Could you check a few things on this model? Use its own coordinates, in mm. Face numbers are marked on the shaded views. A direction names the side the tool comes from. Round coordinates to 2 decimals unless told otherwise and drop trailing zeros. Write each loop counter-clockwise with the first axis right and the second up, starting at its lowest first coordinate (ties: lowest second). Pieces come first, ordered by that corner, then holes. Notation, with made-up numbers: (48, 87.5) -> (102, 87.5) arc R13 ccw to (102, 105.5) -> close; hole circle Ø8 at (44, -27). An arc over 180 degrees is marked (long way). Answer as CSV lines item,"result". Start each with the question number.
Q1. Imagine slicing it at C-C on y = -17. Please give me the cut outline in (x, z), and give its area (3 significant figures).
Q2. Imagine slicing it at B-B on x = 4.5. Please give me the cut outline in (y, z).
Q3. If we mould it in two halves opening along Y, with no side actions, what happens to the marked faces 3, 4 and 5? For each: pulls with the +Y half, pulls with the -Y half, needs draft (parallel to the pull), parting line crosses it, or undercut.
Q4. If I drill on line 1 (X direction, y = -11, z = 2.4); line 2 (Y direction, x = -5, z = 2.25); line 3 (Y direction, x = 7.25, z = 0.7), over which ranges is the centre line in solid material (lowest first)? Write a range as [from, to].
Q5. For the marked faces 1 and 2, which set-ups out of +Z, -Z, +X, -X, +Y, -Y let a thin tool reach every point of the face, with its end or its side?
Q6. Imagine slicing it at D-D on x = -5.5. Please give me the cut outline in (y, z), and give its area (3 significant figures).
Q7. Imagine slicing it at A-A on y = -12.75. Please give me the cut outline in (x, z), and give its area (3 significant figures).
Q8. Will these pins go through, and if not, where does the flat tip stop? pin 1 Ø1 at (x, z) = (2, 1.5) entering from +Y; pin 2 Ø1.2 at (y, z) = (-18.5, 0.5) entering from +X; pin 3 Ø1.2 at (y, z) = (-17.5, 1.5) entering from -X.
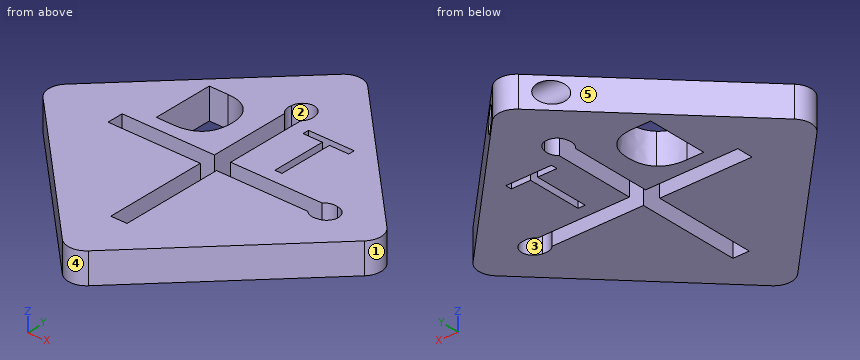
from build123d import *

# Parameters (mm, degrees)
F1_DEPTH = 2.5
F2_R     = 0.85
F3_DEPTH = 12.5


with BuildPart() as f1:
    # F0 (on Top) → F1 (new body)
    with BuildSketch(Plane.XY):
        with BuildLine():
            Line((13.081475452, -13.081475452), (1.0606601718, -1.0606601718))
            ThreePointArc((1.0606601718, -1.0606601718), (0, -0.6213203436), (-1.0606601718, -1.0606601718))
            Line((-1.0606601718, -1.0606601718), (-13.081475452, -13.081475452))
            ThreePointArc((-13.081475452, -13.081475452), (-13.5208152802, -14.1421356237), (-13.081475452, -15.2027957955))
            Line((-13.081475452, -15.2027957955), (-1.0606601718, -27.2236110757))
            ThreePointArc((-1.0606601718, -27.2236110757), (0, -27.6629509039), (1.0606601718, -27.2236110757))
            Line((1.0606601718, -27.2236110757), (13.081475452, -15.2027957955))
            ThreePointArc((13.081475452, -15.2027957955), (13.5208152802, -14.1421356237), (13.081475452, -13.081475452))
        make_face()
        with BuildLine():
            add(Edge.make_bspline(
                [(-2.95422167, -8.1059920208), (-2.3134881631, -8.7467255278), (-2.3134881631, -9.8968991389)],
                knots=[0, 0, 0, 1, 1, 1], degree=2))
            add(Edge.make_bspline(
                [(-2.3134881631, -9.8968991389), (-2.3134881631, -11.1241126806), (-2.9797208019, -11.7735267431)],
                knots=[0, 0, 0, 1, 1, 1], degree=2))
            add(Edge.make_bspline(
                [(-2.9797208019, -11.7735267431), (-3.6459534408, -12.4229408056), (-4.8970385103, -12.4229408056)],
                knots=[0, 0, 0, 1, 1, 1], degree=2))
            Line((-4.8970385103, -12.4229408056), (-6.2707364269, -12.4229408056))
            Line((-6.2707364269, -12.4229408056), (-6.2707364269, -7.4652585139))
            Line((-6.2707364269, -7.4652585139), (-4.7516392047, -7.4652585139))
            add(Edge.make_bspline(
                [(-4.7516392047, -7.4652585139), (-3.5949551769, -7.4652585139), (-2.95422167, -8.1059920208)],
                knots=[0, 0, 0, 1, 1, 1], degree=2))
        make_face(mode=Mode.SUBTRACT)
        with BuildLine():
            Line((-8.1334756687, -14.8039748892), (-8.1334756687, -13.4802963582))
            Line((-8.1334756687, -13.4802963582), (-0.6236797201, -13.4802963582))
            Line((-0.6236797201, -13.4802963582), (-0.6236797201, -6.9198086858))
            ThreePointArc((-0.6236797201, -6.9198086858), (-0.9032194318, -6.4583786209), (-0.9135835525, -5.9189782686))
            ThreePointArc((-0.9135835525, -5.9189782686), (0.0168397474, -5.0141534426), (0.9868078824, -5.876451129))
            ThreePointArc((0.9868078824, -5.876451129), (0.9900106564, -6.4384308628), (0.6999988109, -6.9198086858))
            Line((0.6999988109, -6.9198086858), (0.6999988109, -13.4802963582))
            Line((0.6999988109, -13.4802963582), (8.1334756687, -13.4802963582))
            ThreePointArc((8.1334756687, -13.4802963582), (8.5949057336, -13.2007566465), (9.134306086, -13.1903925258))
            ThreePointArc((9.134306086, -13.1903925258), (10.0391309119, -14.1208158258), (9.1768332255, -15.0907839607))
            ThreePointArc((9.1768332255, -15.0907839607), (8.6148534917, -15.0939867347), (8.1334756687, -14.8039748892))
            Line((8.1334756687, -14.8039748892), (0.6999988109, -14.8039748892))
            Line((0.6999988109, -14.8039748892), (0.6999988109, -23.1867600232))
            Line((0.6999988109, -23.1867600232), (-0.6236797201, -23.1867600232))
            Line((-0.6236797201, -23.1867600232), (-0.6236797201, -14.8039748892))
            Line((-0.6236797201, -14.8039748892), (-8.1334756687, -14.8039748892))
        make_face(mode=Mode.SUBTRACT)
        Polygon((3.9598674141, -7.9774117573), (3.9598674141, -12.4229412712), (3.3836955391, -12.4229412712), (3.3836955391, -7.9774117573), (1.813600053, -7.9774117573), (1.813600053, -7.4652589795), (5.5299629002, -7.4652589795), (5.5299629002, -7.9774117573), align=None, mode=Mode.SUBTRACT)
    extrude(amount=F1_DEPTH)

    # F2 (on Right) → F3 (cut, symmetric)
    with BuildSketch(Plane.YZ):
        with Locations((-2.4908210296, 1.292226194)):
            Circle(F2_R)
    extrude(amount=F3_DEPTH, both=True, mode=Mode.SUBTRACT)


solid = f1.part
Checks:
1,outline,"(-11.28, 0) -> (-0.62, 0) -> (-0.62, 2.5) -> (-11.28, 2.5) -> close; (0.7, 0) -> (11.28, 0) -> (11.28, 2.5) -> (0.7, 2.5) -> close"
1,area,"53.1 mm^2"
2,outline,"(-23.78, 0) -> (-14.8, 0) -> (-14.8, 2.5) -> (-23.78, 2.5) -> close; (-13.48, 0) -> (-7.98, 0) -> (-7.98, 2.5) -> (-13.48, 2.5) -> close; (-7.47, 0) -> (-4.5, 0) -> (-4.5, 2.5) -> (-7.47, 2.5) -> close"
3,face 3,"undercut"
3,face 4,"pulls with the -Y half"
3,face 5,"pulls with the +Y half"
4,line 1,"[-11, -6.27], [-2.49, -0.62], [0.7, 3.38], [3.96, 11]"
4,line 2,"[-23.28, -14.8], [-13.48, -12.42], [-7.47, -5]"
4,line 3,"[-21.03, -14.8], [-13.48, -7.25]"
5,face 1,"+Z, -Z, +X"
5,face 2,"+Z, -Z"
6,outline,"(-22.78, 0) -> (-14.8, 0) -> (-14.8, 2.5) -> (-22.78, 2.5) -> close; (-13.48, 0) -> (-12.42, 0) -> (-12.42, 2.5) -> (-13.48, 2.5) -> close; (-7.47, 0) -> (-5.5, 0) -> (-5.5, 2.5) -> (-7.47, 2.5) -> close"
6,area,"27.5 mm^2"
7,outline,"(-12.75, 0) -> (-0.62, 0) -> (-0.62, 2.5) -> (-12.75, 2.5) -> close; (0.7, 0) -> (12.75, 0) -> (12.75, 2.5) -> (0.7, 2.5) -> close"
7,area,"60.4 mm^2"
8,pin 1,"y = -1.5"
8,pin 2,"x = 10.38"
8,pin 3,"x = -11.38"
